```python
from build123d import *

# Parameters (mm, degrees)
SKETCH_1_W               = 90
SKETCH_1_H               = 30
EXTRUDE_1_DEPTH          = 5
SKETCH_2_W               = 16.25
SKETCH_2_H               = 30
EXTRUDE_2_DEPTH          = 3.5
CUT_EXTRUDE_1_DEPTH      = 49.189729196
CUT_EXTRUDE_1_DEPTH_BACK = 49.189729196
SKETCH_3_R               = 2.9
CHAMFER_1_SIZE           = 1
CUT_EXTRUDE_2_DEPTH      = 48.696960071
CUT_EXTRUDE_2_DEPTH_BACK = 3
SKETCH_4_R               = 9
CHAMFER_2_SIZE           = 1
CUT_EXTRUDE_3_DEPTH      = 48.877447718
CUT_EXTRUDE_3_DEPTH_BACK = 48.877447718
SKETCH_5_R               = 5
CHAMFER_3_SIZE           = 1


with BuildPart() as part:
    # 草图1 → 凸台-拉伸1 (new body)
    with BuildSketch(Plane.XY):
        Rectangle(SKETCH_1_W, SKETCH_1_H)
    extrude(amount=EXTRUDE_1_DEPTH)

    # 草图2 → 凸台-拉伸2 (add)
    with BuildSketch(Plane.XY.offset(5)):
        with Locations((36.875, 0)):
            Rectangle(SKETCH_2_W, SKETCH_2_H)
        with Locations((-36.875, 0)):
            Rectangle(SKETCH_2_W, SKETCH_2_H)
    extrude(amount=EXTRUDE_2_DEPTH)

    # 草图3 → 切除-拉伸1 (cut, two sides: drawn at the far end of the back side and taken through both)
    with BuildSketch(Plane(origin=(0, 0, 0), x_dir=(-1, 0, 0), z_dir=(0, 0, -1)).offset(-CUT_EXTRUDE_1_DEPTH_BACK)):
        with Locations((34, 0)):
            Circle(SKETCH_3_R)
        with Locations((-34, 0)):
            Circle(SKETCH_3_R)
    extrude(amount=CUT_EXTRUDE_1_DEPTH + CUT_EXTRUDE_1_DEPTH_BACK, mode=Mode.SUBTRACT)

    # 倒角1
    chamfer_1_edges = [part.edges().sort_by_distance(p)[0] for p in [
        (-31.1, 0, 0),
        (36.9, 0, 0),
        (0, 15, 0),
        (45, 0, 0),
        (0, -15, 0),
        (-45, 0, 0),
    ]]
    chamfer(chamfer_1_edges, length=CHAMFER_1_SIZE)

    # 草图4 → 切除-拉伸2 (cut, two sides: drawn at the far end of the back side and taken through both)
    with BuildSketch(Plane.XY.offset(5).offset(-CUT_EXTRUDE_2_DEPTH_BACK)):
        Circle(SKETCH_4_R)
    extrude(amount=CUT_EXTRUDE_2_DEPTH + CUT_EXTRUDE_2_DEPTH_BACK, mode=Mode.SUBTRACT)

    # 倒角2
    chamfer_2_edges = [part.edges().sort_by_distance(p)[0] for p in [
        (-9, 0, 5),
    ]]
    chamfer(chamfer_2_edges, length=CHAMFER_2_SIZE)

    # 草图5 → 切除-拉伸3 (cut, two sides: drawn at the far end of the back side and taken through both)
    with BuildSketch(Plane.XY.offset(2).offset(-CUT_EXTRUDE_3_DEPTH_BACK)):
        Circle(SKETCH_5_R)
    extrude(amount=CUT_EXTRUDE_3_DEPTH + CUT_EXTRUDE_3_DEPTH_BACK, mode=Mode.SUBTRACT)

    # 倒角3
    chamfer_3_edges = [part.edges().sort_by_distance(p)[0] for p in [
        (-5, 0, 2),
        (-5, 0, 0),
    ]]
    chamfer(chamfer_3_edges, length=CHAMFER_3_SIZE - 0.0001)  # a hair under: the kernel refuses the full size


solid = part.part
```
Source: CAD feature listing. Evaluate the final solid. Frame: model axes, mm. A direction names the side the tool comes from. Coordinates: 2 decimals unless noted, no trailing zeros. Write each loop counter-clockwise with the first axis right and the second up, starting at its lowest first coordinate (ties: lowest second). Pieces come first, ordered by that corner, then holes. Notation, with made-up numbers: (-33, -35.75) -> (-15, -35.75) arc R23 cw to (-15, -20.75) -> close; hole circle Ø11 at (-24.5, -7.5). An arc over 180 degrees is marked (long way). Return JSON: item names as keys, results as strings. Group by question number.
1) Section query C-C, the plane y = 0. State how many separate pieces and enclosed holes the cut face has, plus the area to 3 significant figures.
2) Contact query for flat-ended pins moving along their axis: P1, Ø2, axis at x = 7.5, y = 6, coming from the +Z side; P2, Ø4.5, axis at x = -34, y = 0, coming from the -Z side (1 decimal). Output: stop coordinate, or through.
3) Ray query, line 1 along X through (y, z) = (0, 3); line 2 along Y through (x, z) = (34, 6.75); line 3 along X through (y, z) = (7, 7). Return the intervals inside material, ascending.
4) Section query B-B, the plane z = 6.75. Return loops of the section in (x, y), plus the area to 3 significant figures.
5) Set-up query: faces 1 (the face through (-28.75, 0, 7)), 2 (the face through (-1.172, 8.923, 2.986)), 3 (the face through (-45, 0, 5)). Return all of +Z, -Z, +X, -X, +Y, -Y with unobstructed straight access to the full face (end or side cutting, diameter ignored); none if empty.
6) Section query A-A, the plane x = -34. Return loops of the section in (y, z).
7) Mould query, pull axis Y, two halves, no side actions, for faces 4 (the face through (-0.6, 6.4, 0)), 5 (the face through (-36.766, 0.871, 4.803)), 6 (the face through (-1, 15, 4)), 7 (the face through (-1, -15, 4)). Classes: +Y half, -Y half, draft (parallel to the pull), parting line (faces both ways), or undercut.
From the geometry:
{
 "1": {"separate pieces": "4", "enclosed holes": "0", "area": "385 mm²"},
 "2": {"P1": "z = 5", "P2": "through"},
 "3": {"line 1": "-45 to -36.9, -31.1 to -9, 9 to 31.1, 36.9 to 45", "line 2": "-15 to -2.9, 2.9 to 15", "line 3": "-45 to -28.75, 28.75 to 45"},
 "4": {"outline": "(-45, -15) -> (-28.75, -15) -> (-28.75, 15) -> (-45, 15) -> close; (28.75, -15) -> (45, -15) -> (45, 15) -> (28.75, 15) -> close; hole circle Ø5.8 at (-34, 0); hole circle Ø5.8 at (34, 0)", "area": "922 mm²"},
 "5": {"face 1": "+Z, +Y, -Y", "face 2": "+Z", "face 3": "+Z, -Z, -X, +Y, -Y"},
 "6": {"outline": "(-15, 1) -> (-14, 0) -> (-3.9, 0) -> (-2.9, 1) -> (-2.9, 8.5) -> (-15, 8.5) -> close; (2.9, 1) -> (3.9, 0) -> (14, 0) -> (15, 1) -> (15, 8.5) -> (2.9, 8.5) -> close"},
 "7": {"face 4": "draft", "face 5": "undercut", "face 6": "+Y half", "face 7": "-Y half"}
}
